Here's how the part is built. I have some questions about the finished solid (model axes, mm). Face numbers are marked on the shaded views. A direction names the side the tool comes from. Coordinates: 2 decimals unless noted, no trailing zeros. Order: outer loops, then holes, each group sorted by start corner. A loop starts at its lowest first (then second) coordinate and runs counter-clockwise, first axis right, second up. Notation, with made-up numbers: (46, 2.25) - (60, 2.25) arc R21 cw to (60, 8.25) - close; hole circle Ø2 at (-18, 89). An arc over 180 degrees is marked (long way). Answer in a Markdown table with one row per item. Add a question column.
Item 1: I want a section at A-A (z = 1). Please give me the cut outline in (x, y), plus the area to 3 significant figures.
Item 2: I want a section at B-B (x = -0.75). Please give me the cut outline in (y, z).
Item 3: If I drill on line 1 along Z through (x, y) = (-0.5, 4.25); line 2 along Y through (x, z) = (-1, -1.3); line 3 along X through (y, z) = (6.75, -1.05), over which ranges is the centre line in solid material (lowest first)? Write a range as from..to.
Item 4: I want a section at C-C (z = -1.5). Please give me the cut outline in (x, y), plus the area to 3 significant figures.
Item 5: Will these pins go through, and if not, where does the flat tip stop? pin 1 Ø1.2 at (x, y) = (-0.5, 6) entering from +Z; pin 2 Ø1 at (x, y) = (1, 7) entering from -Z; pin 3 Ø1.5 at (x, y) = (2.5, 5.5) entering from -Z.
Item 6: On a 3-axis mill with a long thin cutter (end or side, diameter ignored), from which of +Z, -Z, +X, -X, +Y, -Y can I reach the whole of each face in a straight line? I mean the marked faces 1, 2, 3 and 4. Say none if no direction works.
Item 7: I want a section at D-D (x = 3). Please give me the cut outline in (y, z), plus the area to 3 significant figures.
```python
from build123d import *

# Parameters (mm, degrees)
SKETCH1_W           = 7
SKETCH1_H           = 5
BOSS_EXTRUDE1_DEPTH = 3
SKETCH2_W           = 4.4
SKETCH2_H           = 2.4
BOSS_EXTRUDE2_DEPTH = 5
FILLET1_R           = 1


with BuildPart() as part:
    # Sketch1 → Boss-Extrude1 (new body)
    with BuildSketch(Plane(origin=(0, 0, 0), x_dir=(1, 0, 0), z_dir=(0, 1, 0))):
        Rectangle(SKETCH1_W, SKETCH1_H)
    extrude(amount=BOSS_EXTRUDE1_DEPTH)

    # Sketch2 → Boss-Extrude2 (add)
    with BuildSketch(Plane(origin=(0, 3, 0), x_dir=(1, 0, 0), z_dir=(0, 1, 0))):
        Rectangle(SKETCH2_W, SKETCH2_H)
    extrude(amount=BOSS_EXTRUDE2_DEPTH)

    # Fillet1
    fillet1_edges = [part.edges().sort_by_distance(p)[0] for p in [
        (2.2, 5.5, 1.2),
        (2.2, 5.5, -1.2),
        (-2.2, 5.5, -1.2),
        (-2.2, 5.5, 1.2),
    ]]
    fillet(fillet1_edges, radius=FILLET1_R)


solid = part.part
```
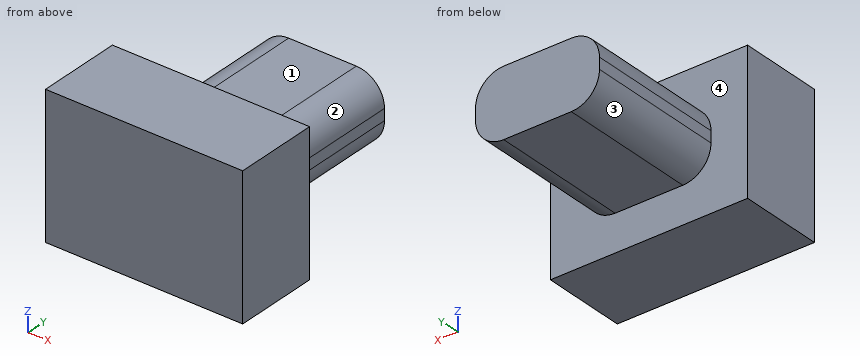
Values follow:
| question | item | result |
|---|---|---|
| 1 | outline | (-3.5, 0) - (3.5, 0) - (3.5, 3) - (1.8, 3) - (1.8, 8) - (-1.8, 8) - (-1.8, 3) - (-3.5, 3) - close |
| 1 | area | 39.0 mm^2 |
| 2 | outline | (0, -2.5) - (3, -2.5) - (3, -1.2) - (8, -1.2) - (8, 1.2) - (3, 1.2) - (3, 2.5) - (0, 2.5) - close |
| 3 | line 1 | z = -1.2..1.2 |
| 3 | line 2 | y = 0..3 |
| 3 | line 3 | x = -1.73..1.73 |
| 4 | outline | (-3.5, 0) - (3.5, 0) - (3.5, 3) - (-3.5, 3) - close |
| 4 | area | 21.0 mm^2 |
| 5 | pin 1 | stops at z = 1.2 |
| 5 | pin 2 | stops at z = -1.2 |
| 5 | pin 3 | stops at z = -1.04 |
| 6 | face 1 | +Z, +X, -X, +Y |
| 6 | face 2 | +Z, +X, +Y |
| 6 | face 3 | -Z, -X, +Y |
| 6 | face 4 | +Y |
| 7 | outline | (0, -2.5) - (3, -2.5) - (3, 2.5) - (0, 2.5) - close |
| 7 | area | 15.0 mm^2 |
